Work out the finished part from the listing and answer in its coordinate system (mm). Round coordinates to 2 decimals unless told otherwise and drop trailing zeros. Loops run counter-clockwise (first coordinate to the right, second up) from the corner with the lowest first, then second, coordinate; pieces in that order, holes last. Notation, with made-up numbers: (62, 85.5) -> (83, 85.5) arc R26 cw to (83, 123.5) -> close; hole circle Ø3 at (16.25, 30). An arc over 180 degrees is marked (long way). Write item = value, one per line. Start each with the question number.
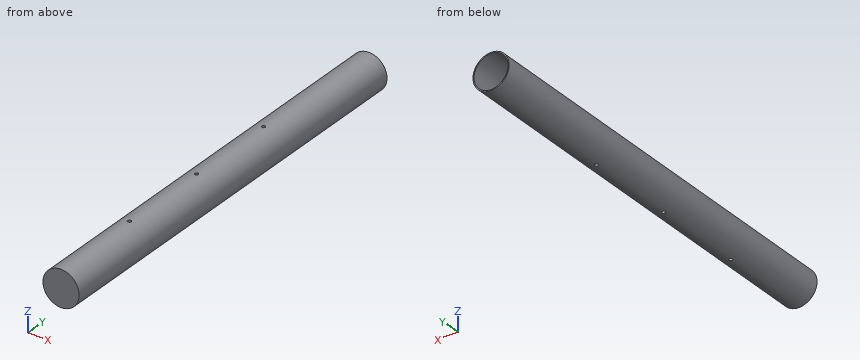
```python
from build123d import *
from build123d.topology import SkipClean

# Parameters (mm, degrees)
SKETCH1_R               = 10.3
BOSS_EXTRUDE1_DEPTH     = 210
BOSS_EXTRUDE3_START     = -2
SKETCH1_4_R             = 10.3
SKETCH1_4_R_2           = 9.7
SKETCH1_4_R_3           = 6.25
BOSS_EXTRUDE3_DEPTH     = 2
BOSS_EXTRUDE2_START     = 210
SKETCH1_3_R             = 10.3
SKETCH1_3_R_2           = 9.7
BOSS_EXTRUDE2_DEPTH     = 29
FILLET1_R               = 2
CUT_EXTRUDE1_REACH      = 242.107
CUT_EXTRUDE1_END_RADIUS = 6.25
SKETCH3_R               = 1
CIRPATTERN1_COUNT       = 2


with BuildPart() as part:
    # Sketch1 → Boss-Extrude1 (new body)
    with BuildSketch(Plane(origin=(0, 0, 0), x_dir=(1, 0, 0), z_dir=(0, 1, 0))):
        with Locations(Location((0, 0, 0), (0, 0, 270))):
            Circle(SKETCH1_R)
        with BuildLine():
            Line((6.16948134, 1), (9.648315915, 1))
            ThreePointArc((9.648315915, 1), (9.7, 0), (9.648315915, -1))
            Line((9.648315915, -1), (6.16948134, -1))
            ThreePointArc((6.16948134, -1), (0, -6.25), (-6.16948134, -1))
            Line((-6.16948134, -1), (-9.648315915, -1))
            ThreePointArc((-9.648315915, -1), (-9.7, 0), (-9.648315915, 1))
            Line((-9.648315915, 1), (-6.16948134, 1))
            ThreePointArc((-6.16948134, 1), (0, 6.25), (6.16948134, 1))
        make_face(mode=Mode.SUBTRACT)
    extrude(amount=BOSS_EXTRUDE1_DEPTH)

    # Sketch1<4> → Boss-Extrude3 (add)
    # profile 1 of 6: a face of its own
    with BuildSketch(Plane(origin=(0, 0, 0), x_dir=(1, 0, 0), z_dir=(0, 1, 0)).offset(BOSS_EXTRUDE3_START)):
        with Locations(Location((0, 0, 0), (0, 0, 270))):
            Circle(SKETCH1_4_R)
        Circle(SKETCH1_4_R_2, mode=Mode.SUBTRACT)
    # profile 2 of 6: a face of its own
    with BuildSketch(Plane(origin=(0, 0, 0), x_dir=(1, 0, 0), z_dir=(0, 1, 0)).offset(BOSS_EXTRUDE3_START)):
        with BuildLine():
            ThreePointArc((9.648315915, 1), (0, 9.7), (-9.648315915, 1))
            Line((-9.648315915, 1), (-6.16948134, 1))
            ThreePointArc((-6.16948134, 1), (0, 6.25), (6.16948134, 1))
            Line((6.16948134, 1), (9.648315915, 1))
        make_face()
    # profile 3 of 6: a face of its own
    with BuildSketch(Plane(origin=(0, 0, 0), x_dir=(1, 0, 0), z_dir=(0, 1, 0)).offset(BOSS_EXTRUDE3_START)):
        with BuildLine():
            ThreePointArc((9.7, 0), (9.687070362, 0.500667366), (9.648315915, 1))
            Line((9.648315915, 1), (6.16948134, 1))
            ThreePointArc((6.16948134, 1), (6.229837814, 0.501618195), (6.25, 0))
            ThreePointArc((6.25, 0), (6.229837814, -0.501618195), (6.16948134, -1))
            Line((6.16948134, -1), (9.648315915, -1))
            ThreePointArc((9.648315915, -1), (9.687070362, -0.500667366), (9.7, 0))
        make_face()
    # profile 4 of 6: a face of its own
    with BuildSketch(Plane(origin=(0, 0, 0), x_dir=(1, 0, 0), z_dir=(0, 1, 0)).offset(BOSS_EXTRUDE3_START)):
        with BuildLine():
            Line((-6.16948134, -1), (-9.648315915, -1))
            ThreePointArc((-9.648315915, -1), (0, -9.7), (9.648315915, -1))
            Line((9.648315915, -1), (6.16948134, -1))
            ThreePointArc((6.16948134, -1), (0, -6.25), (-6.16948134, -1))
        make_face()
    # profile 5 of 6: a face of its own
    with BuildSketch(Plane(origin=(0, 0, 0), x_dir=(1, 0, 0), z_dir=(0, 1, 0)).offset(BOSS_EXTRUDE3_START)):
        Circle(SKETCH1_4_R_3)
    # profile 6 of 6: a face of its own
    with BuildSketch(Plane(origin=(0, 0, 0), x_dir=(1, 0, 0), z_dir=(0, 1, 0)).offset(BOSS_EXTRUDE3_START)):
        with BuildLine():
            Line((-6.16948134, 1), (-9.648315915, 1))
            ThreePointArc((-9.648315915, 1), (-9.7, 0), (-9.648315915, -1))
            Line((-9.648315915, -1), (-6.16948134, -1))
            ThreePointArc((-6.16948134, -1), (-6.25, 0), (-6.16948134, 1))
        make_face()
    extrude(amount=BOSS_EXTRUDE3_DEPTH)

    # Sketch1<3> → Boss-Extrude2 (add)
    with SkipClean():  # the faces are left unmerged after this step: merging them gives an invalid solid
        with BuildSketch(Plane(origin=(0, 0, 0), x_dir=(1, 0, 0), z_dir=(0, 1, 0)).offset(BOSS_EXTRUDE2_START)):
            with Locations(Location((0, 0, 0), (0, 0, 270))):
                Circle(SKETCH1_3_R)
            with Locations(Location((0, 0, 0), (0, 0, 174.082705248))):
                Circle(SKETCH1_3_R_2, mode=Mode.SUBTRACT)
        extrude(amount=BOSS_EXTRUDE2_DEPTH)

    # Fillet1
    fillet1_edges = [part.edges().sort_by_distance(p)[0] for p in [
        (6.16948134, 105, 1),
        (6.16948134, 105, -1),
        (-6.16948134, 105, -1),
        (-6.16948134, 105, 1),
    ]]
    fillet(fillet1_edges, radius=FILLET1_R)

    # Cut-Extrude1: up to this cylinder (the profile starts outside it)
    with SkipClean():  # the faces are left unmerged after this step: merging them gives an invalid solid
        cut_extrude1_end = Plane(origin=(0, 104, 0), z_dir=(0, -1, 0)) * Cylinder(CUT_EXTRUDE1_END_RADIUS, 602.714, mode=Mode.PRIVATE)
        # Sketch3 → Cut-Extrude1 (cut, up to the surface)
        with BuildSketch(Plane.XY.offset(10.3), mode=Mode.PRIVATE) as cut_extrude1_sk1:
            with BuildLine():
                ThreePointArc((1, 104), (0.707106781, 104.707106781), (0, 105))
                Line((0, 105), (0, 103))
                ThreePointArc((0, 103), (0.707106781, 103.292893219), (1, 104))
            make_face()
        cut_extrude1_tool1 = extrude(cut_extrude1_sk1.sketch, amount=-CUT_EXTRUDE1_REACH, mode=Mode.PRIVATE) - cut_extrude1_end
        # Sketch3 → Cut-Extrude1 (cut, up to the surface)
        with BuildSketch(Plane.XY.offset(10.3), mode=Mode.PRIVATE) as cut_extrude1_sk2:
            with BuildLine():
                Line((0, 103), (0, 105))
                ThreePointArc((0, 105), (-1, 104), (0, 103))
            make_face()
        cut_extrude1_tool2 = extrude(cut_extrude1_sk2.sketch, amount=-CUT_EXTRUDE1_REACH, mode=Mode.PRIVATE) - cut_extrude1_end
        # Sketch3 → Cut-Extrude1 (cut, up to the surface)
        with BuildSketch(Plane.XY.offset(10.3), mode=Mode.PRIVATE) as cut_extrude1_sk3:
            with BuildLine():
                ThreePointArc((1, 104), (0.707106781, 104.707106781), (0, 105))
                Line((0, 105), (0, 103))
                ThreePointArc((0, 103), (0.707106781, 103.292893219), (1, 104))
            make_face()
        cut_extrude1_tool3 = extrude(cut_extrude1_sk3.sketch, amount=-CUT_EXTRUDE1_REACH, mode=Mode.PRIVATE) - cut_extrude1_end
        # Sketch3 → Cut-Extrude1 (cut, up to the surface)
        with BuildSketch(Plane.XY.offset(10.3), mode=Mode.PRIVATE) as cut_extrude1_sk4:
            with BuildLine():
                Line((0, 103), (0, 105))
                ThreePointArc((0, 105), (-1, 104), (0, 103))
            make_face()
        cut_extrude1_tool4 = extrude(cut_extrude1_sk4.sketch, amount=-CUT_EXTRUDE1_REACH, mode=Mode.PRIVATE) - cut_extrude1_end
        # Sketch3 → Cut-Extrude1 (cut, up to the surface)
        with BuildSketch(Plane.XY.offset(10.3), mode=Mode.PRIVATE) as cut_extrude1_sk5:
            with Locations((0, 156.5)):
                Circle(SKETCH3_R)
        cut_extrude1_tool5 = extrude(cut_extrude1_sk5.sketch, amount=-CUT_EXTRUDE1_REACH, mode=Mode.PRIVATE) - cut_extrude1_end
        # Sketch3 → Cut-Extrude1 (cut, up to the surface)
        with BuildSketch(Plane.XY.offset(10.3), mode=Mode.PRIVATE) as cut_extrude1_sk6:
            with Locations((0, 51.5)):
                Circle(SKETCH3_R)
        cut_extrude1_tool6 = extrude(cut_extrude1_sk6.sketch, amount=-CUT_EXTRUDE1_REACH, mode=Mode.PRIVATE) - cut_extrude1_end
        cut_extrude1 = cut_extrude1_tool1.solids().sort_by_distance((0.424413, 104, 10.3))[0] + cut_extrude1_tool2.solids().sort_by_distance((-0.424413, 104, 10.3))[0] + cut_extrude1_tool3.solids().sort_by_distance((0.424413, 104, 10.3))[0] + cut_extrude1_tool4.solids().sort_by_distance((-0.424413, 104, 10.3))[0] + cut_extrude1_tool5.solids().sort_by_distance((0, 156.5, 10.3))[0] + cut_extrude1_tool6.solids().sort_by_distance((0, 51.5, 10.3))[0]
        add(cut_extrude1, mode=Mode.SUBTRACT)

    # CirPattern1: Cut-Extrude1 ×2 about axis
    with SkipClean():  # the faces are left unmerged after this step: merging them gives an invalid solid
        cirpattern1_axis = Axis((0, 210, 0), (0, -1, 0))
        for i in range(1, CIRPATTERN1_COUNT):
            add(cut_extrude1.rotate(cirpattern1_axis, i * 360 / CIRPATTERN1_COUNT), mode=Mode.SUBTRACT)


solid = part.part
```
Item 1: Flat-ended cylindrical pins translate along their axes: pin 1 (5 mm diameter, centred on x = -2, z = 6, fed in from +Y); pin 2 (3 mm diameter, centred on x = -0.5, z = 2.5, fed in from +Y); pin 3 (0.6 mm diameter, centred on x = -9, y = 87, fed in from +Z). Find the tip coordinate at first contact, or state that the pin passes through.
Item 2: Section B-B (y = 218) is taken. Determine the outline of the cut face in (x, z).
Item 3: Section A-A (y = 113) is taken. Determine the outline of the cut face in (x, z), then the cut area to 3 significant figures.
Item 4: Find the intervals of material crossed by line 1 along Y through (x, z) = (0, 8.55); line 2 along Y through (x, z) = (-0.5, 7.25); line 3 along X through (y, z) = (156.5, -8.25), in increasing order. Write a range as [from, to].
Worked answers:
q1.pin_1 = 210
q1.pin_2 = 0
q1.pin_3 = 5.51
q2.outline = circle Ø20.6 at (0, 0); hole circle Ø19.4 at (0, 0)
q3.outline = circle Ø20.6 at (0, 0); hole (-9.65, -1) -> (-7.69, -1) arc R2 cw to (-5.82, -2.27) arc R6.25 ccw to (5.82, -2.27) arc R2 cw to (7.69, -1) -> (9.65, -1) arc R9.7 ccw to (9.65, 1) -> (7.69, 1) arc R2 cw to (5.82, 2.27) arc R6.25 ccw to (-5.82, 2.27) arc R2 cw to (-7.69, 1) -> (-9.65, 1) arc R9.7 ccw to start
q3.area = 195 mm2
q4.line_1 = [-2, 50.5], [52.5, 103], [105, 155.5], [157.5, 210]
q4.line_2 = [-2, 50.63], [52.37, 103.13], [104.87, 155.63], [157.37, 210]
q4.line_3 = [-6.17, -1], [1, 6.17]
